Verification items for the finished model (mm, model axes). A direction names the side the tool comes from. Give positions to 0.01 mm unless a question says otherwise; leave off trailing zeros. Write each loop counter-clockwise with the first axis right and the second up, starting at its lowest first coordinate (ties: lowest second). Pieces come first, ordered by that corner, then holes.
from build123d import *

# Parameters (mm, degrees)
BOSS_EXTRUDE1_DEPTH = 24
SKETCH2_R           = 1
CUT_EXTRUDE1_DEPTH  = 13


with BuildPart() as part:
    # Sketch1 → Boss-Extrude1 (new body)
    with BuildSketch(Plane.XY):
        with BuildLine():
            Line((-0.9, 2.170829335), (-0.9, 0.9))
            Line((-0.9, 0.9), (-2.170829335, 0.9))
            ThreePointArc((-2.170829335, 0.9), (-2.35, 0), (-2.170829335, -0.9))
            Line((-2.170829335, -0.9), (-0.9, -0.9))
            Line((-0.9, -0.9), (-0.9, -2.170829335))
            ThreePointArc((-0.9, -2.170829335), (0, -2.35), (0.9, -2.170829335))
            Line((0.9, -2.170829335), (0.9, -0.9))
            Line((0.9, -0.9), (2.170829335, -0.9))
            ThreePointArc((2.170829335, -0.9), (2.35, 0), (2.170829335, 0.9))
            Line((2.170829335, 0.9), (0.9, 0.9))
            Line((0.9, 0.9), (0.9, 2.170829335))
            ThreePointArc((0.9, 2.170829335), (0, 2.35), (-0.9, 2.170829335))
        make_face()
    extrude(amount=BOSS_EXTRUDE1_DEPTH)

    # Sketch2 → Cut-Extrude1 (cut)
    with BuildSketch(Plane.XY.offset(24)):
        Circle(SKETCH2_R)
    extrude(amount=-CUT_EXTRUDE1_DEPTH, mode=Mode.SUBTRACT)


solid = part.part
Item 1: Sectioned sample at B-B on y = 0. Record the cut outline in (x, z).
Answer key:
outline: (-2.35, 0) - (2.35, 0) - (2.35, 24) - (1, 24) - (1, 11) - (-1, 11) - (-1, 24) - (-2.35, 24) - close
Item 2: Scan lines: line 1 along Y through (x, z) = (0, 20.5); line 2 along Y through (x, z) = (1.7, 15.25); line 3 along Z through (x, y) = (-0.65, 0.45). Record each from-to range of solid material in increasing order.
Answer key:
line 1: y = -2.35 to -1, 1 to 2.35
line 2: y = -0.9 to 0.9
line 3: z = 0 to 11
Item 3: Release check for a two-part mould opening along X. For faces 1 (the face through (0, -1, 18)), 2 (the face through (0, 0, 11)), 3 (the face through (-0.9, -2, 12)), 4 (the face through (2, 0.9, 12)) record: released by +X, released by -X, zero draft, split by the parting line, or undercut.
Answer key:
face 1: undercut
face 2: undercut
face 3: released by -X
face 4: zero draft
Item 4: Set-up check for faces 5 (the face through (-2, 0.9, 12)), 6 (the face through (2, -0.9, 12)), 7 (the face through (-2.35, 0.01, 11.83)), 8 (the face through (0.9, 2, 12)), 9 (the face through (-2, -0.9, 12)): record each of +Z, -Z, +X, -X, +Y, -Y from which the full face is reachable in a straight line by a thin tool's end or side.
Answer key:
face 5: +Z, -Z, -X, +Y
face 6: +Z, -Z, +X, -Y
face 7: +Z, -Z, -X
face 8: +Z, -Z, +X, +Y
face 9: +Z, -Z, -X, -Y
Item 5: Sectioned sample at D-D on z = 7.25. Record the cut outline in (x, y).
Answer key:
outline: (-2.17, -0.9) - (-0.9, -0.9) - (-0.9, -2.17) arc R2.35 ccw to (0.9, -2.17) - (0.9, -0.9) - (2.17, -0.9) arc R2.35 ccw to (2.17, 0.9) - (0.9, 0.9) - (0.9, 2.17) arc R2.35 ccw to (-0.9, 2.17) - (-0.9, 0.9) - (-2.17, 0.9) arc R2.35 ccw to start
Item 6: Depth check by flat-ended pin: pin 1 (0.6 mm diameter, centred on x = 0, y = -0.5, fed in from +Z); pin 2 (1 mm diameter, centred on x = 1.5, z = 11.5, fed in from +Y); pin 3 (2 mm diameter, centred on x = -1.5, z = 6.5, fed in from -Y). Enter the tip coordinate at first touch or a pass-through.
Answer key:
pin 1: stops at z = 11
pin 2: stops at y = 0.9
pin 3: stops at y = -2.3
Item 7: Sectioned sample at A-A on z = 16.5. Record the cut outline in (x, y).
Answer key:
outline: (-2.17, -0.9) - (-0.9, -0.9) - (-0.9, -2.17) arc R2.35 ccw to (0.9, -2.17) - (0.9, -0.9) - (2.17, -0.9) arc R2.35 ccw to (2.17, 0.9) - (0.9, 0.9) - (0.9, 2.17) arc R2.35 ccw to (-0.9, 2.17) - (-0.9, 0.9) - (-2.17, 0.9) arc R2.35 ccw to start; hole circle Ø2 at (0, 0)
